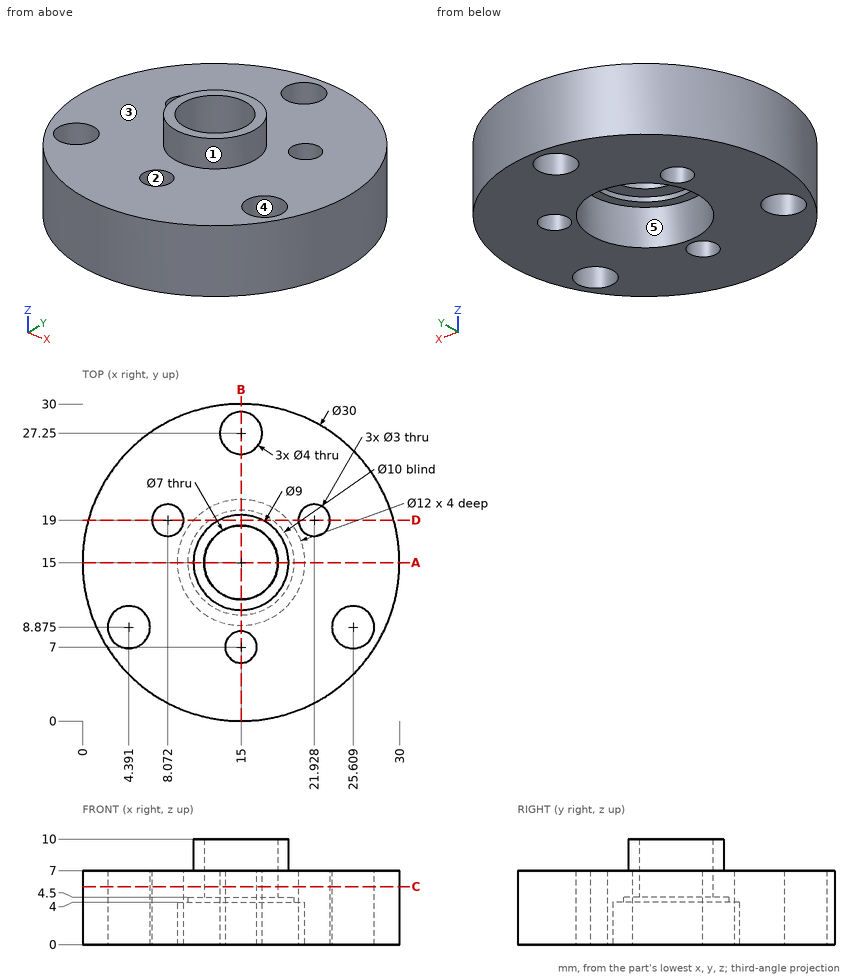
Part print with two shaded views. Sizes in mm from the minimum x, y, z corner. A direction names the side the tool comes from. Round coordinates to 2 decimals unless told otherwise and drop trailing zeros. Order: outer loops, then holes, each group sorted by start corner. A loop starts at its lowest first (then second) coordinate and runs counter-clockwise, first axis right, second up.
(1) Pin check, flat tips, straight feed: pin 1 (5 mm diameter, centred on x = 15.5, y = 13, fed in from -Z); pin 2 (8 mm diameter, centred on x = 25.5, y = 18.5, fed in from +Z); pin 3 (4 mm diameter, centred on x = 9.5, z = 2.5, fed in from +Y). Stop position of each tip, or through.
(2) 3-axis set-ups, long thin cutter, end or side, ignore diameter. For the marked faces 4 and 5: which of +Z, -Z, +X, -X, +Y, -Y reach the whole face in a straight line?
(3) Drill centre lines: line 1 (Y direction, x = 15, z = 4.25); line 2 (Y direction, x = 15, z = 3); line 3 (X direction, y = 19.5, z = 6.5). Where is each one in solid material? Low to high.
(4) Band-saw the part on C-C (z = 5.5). Give the number of separate pieces and of enclosed holes in the cut face.
(5) Band-saw the part on A-A (y = 15). List the corners of the cut face in (x, z), then the cut area to 4 significant figures.
(6) Pull direction Y, two halves, no side cores. Call the marked faces 1, 2 and 3: released by +Y, released by -Y, zero draft, split by the parting line, or undercut.
(7) Band-saw the part on D-D (y = 19). List the corners of the cut face in (x, z).
(8) Band-saw the part on B-B (x = 15). List the corners of the cut face in (y, z).
Verdict:
1. pin 1: stops at z = 4.5
1. pin 2: stops at z = 7
1. pin 3: stops at y = 29.59
2. face 4: +Z, -Z
2. face 5: -Z
3. line 1: y = 0 to 5.5, 8.5 to 10, 20 to 25.25, 29.25 to 30
3. line 2: y = 0 to 5.5, 8.5 to 9, 21 to 25.25, 29.25 to 30
3. line 3: x = 0.69 to 6.66, 9.49 to 20.51, 23.34 to 29.31
4. separate pieces: 1
4. enclosed holes: 7
5. outline: (0, 0) - (9, 0) - (9, 4) - (10, 4) - (10, 4.5) - (11.5, 4.5) - (11.5, 10) - (10.5, 10) - (10.5, 7) - (0, 7) - close; (18.5, 4.5) - (20, 4.5) - (20, 4) - (21, 4) - (21, 0) - (30, 0) - (30, 7) - (19.5, 7) - (19.5, 10) - (18.5, 10) - close
5. area: 145.5 mm2
6. face 1: split by the parting line
6. face 2: undercut
6. face 3: zero draft
7. outline: (0.54, 0) - (6.57, 0) - (6.57, 7) - (0.54, 7) - close; (9.57, 0) - (10.53, 0) - (10.53, 4) - (12, 4) - (12, 4.5) - (18, 4.5) - (18, 4) - (19.47, 4) - (19.47, 0) - (20.43, 0) - (20.43, 7) - (17.06, 7) - (17.06, 10) - (12.94, 10) - (12.94, 7) - (9.57, 7) - close; (23.43, 0) - (29.46, 0) - (29.46, 7) - (23.43, 7) - close
8. outline: (0, 0) - (5.5, 0) - (5.5, 7) - (0, 7) - close; (8.5, 0) - (9, 0) - (9, 4) - (10, 4) - (10, 4.5) - (11.5, 4.5) - (11.5, 10) - (10.5, 10) - (10.5, 7) - (8.5, 7) - close; (18.5, 4.5) - (20, 4.5) - (20, 4) - (21, 4) - (21, 0) - (25.25, 0) - (25.25, 7) - (19.5, 7) - (19.5, 10) - (18.5, 10) - close; (29.25, 0) - (30, 0) - (30, 7) - (29.25, 7) - close
